from build123d import *

# Parameters (mm, degrees)
BOSS_EXTRUDE1_DEPTH                                  = 50.8
CBORE_FOR_1_4_BINDING_HEAD_MACHINE_SCREW_D           = 6.5278
CBORE_FOR_1_4_BINDING_HEAD_MACHINE_SCREW_CBORE_D     = 14.2875
CBORE_FOR_1_4_BINDING_HEAD_MACHINE_SCREW_CBORE_DEPTH = 3.302
CUT_EXTRUDE1_REACH                                   = 73.186
SKETCH4_R                                            = 3.175


with BuildPart() as part:
    # Sketch1 → Boss-Extrude1 (new body)
    with BuildSketch(Plane(origin=(0, 0, 0), x_dir=(0, 0, -1), z_dir=(1, 0, 0))):
        Polygon((0, 0), (0, 29.972), (39.856315031, 29.972), (39.856315031, 25.3111), (8.106315031, 25.3111), (8.106315031, 4.6609), (39.856315031, 4.6609), (39.856315031, 0), align=None)
    extrude(amount=BOSS_EXTRUDE1_DEPTH)

    # CBORE for 1/4 Binding Head Machine Screw1 (through all)
    with Locations(Plane(origin=(0, 0, -8.106315031), x_dir=(-1, 0, 0), z_dir=(0, 0, -1))):
        with Locations((-12.7, 14.986), (-38.1, 14.986)):
            CounterBoreHole(CBORE_FOR_1_4_BINDING_HEAD_MACHINE_SCREW_D / 2, CBORE_FOR_1_4_BINDING_HEAD_MACHINE_SCREW_CBORE_D / 2, CBORE_FOR_1_4_BINDING_HEAD_MACHINE_SCREW_CBORE_DEPTH)

    # Cut-Extrude1: up to this face of the body (flat: up to its plane)
    cut_extrude1_end = Plane(part.part.faces().sort_by_distance((25.4, 29.972, -19.928157515))[0])
    # Sketch4 → Cut-Extrude1 (cut, up to the picked face)
    with BuildSketch(Plane.XZ, mode=Mode.PRIVATE) as cut_extrude1_sk1:
        with Locations(Location((25.4, -29.497789369, 0), (0, 0, 270))):
            Circle(SKETCH4_R)
    cut_extrude1_tool1 = split(extrude(cut_extrude1_sk1.sketch, amount=-CUT_EXTRUDE1_REACH, mode=Mode.PRIVATE), bisect_by=cut_extrude1_end, keep=Keep.BOTH, mode=Mode.PRIVATE)
    # Sketch4 → Cut-Extrude1 (cut, up to the picked face)
    with BuildSketch(Plane.XZ, mode=Mode.PRIVATE) as cut_extrude1_sk2:
        with BuildLine():
            Line((0, 0), (16.880765903, -33.757868641))
            ThreePointArc((16.880765903, -33.757868641), (25.4, -39.022789369), (33.919234097, -33.757868641))
            Line((33.919234097, -33.757868641), (50.8, 0))
            Line((50.8, 0), (50.8, -39.856315031))
            Line((50.8, -39.856315031), (0, -39.856315031))
            Line((0, -39.856315031), (0, 0))
        make_face()
    cut_extrude1_tool2 = split(extrude(cut_extrude1_sk2.sketch, amount=-CUT_EXTRUDE1_REACH, mode=Mode.PRIVATE), bisect_by=cut_extrude1_end, keep=Keep.BOTH, mode=Mode.PRIVATE)
    add(cut_extrude1_tool1.solids().sort_by(Axis((25.4, 0, -29.497789), (0, 1, 0)))[0], mode=Mode.SUBTRACT)
    add(cut_extrude1_tool2.solids().sort_by(Axis((7.862872, 0, -17.167721), (0, 1, 0)))[0], mode=Mode.SUBTRACT)


solid = part.part
Design review of the part built by this model. Coordinates are the model's own, in mm. A direction names the side the tool comes from. Give positions to 0.01 mm unless a question says otherwise; leave off trailing zeros. Loops run counter-clockwise (first coordinate to the right, second up) from the corner with the lowest first, then second, coordinate; pieces in that order, holes last. Notation, with made-up numbers: (37.5, 50.25) -> (47.5, 50.25) arc R13 ccw to (47.5, 72.25) -> close; hole circle Ø3 at (12, -27). An arc over 180 degrees is marked (long way). One line per question, with ' | ' between items. Start each with the question number.
(1) We need section C-C (y = 16). State the section outline as (x, z) points.
(2) Draft analysis for pull direction X (two halves, no side actions). For faces 1 (the face through (47.87, 14.78, -5.86)), 2 (the face through (45.237, 15.3, -6.478)), 3 (the face through (17.97, 19.81, -6.48)), 4 (the face through (25, 25.311, -20)), state which applies: +X half, -X half, draft (parallel to the pull), parting line (faces both ways), or undercut.
(3) For faces 5 (the face through (28.08, 27.61, -31.2)), 6 (the face through (36.6, 11.9, -4.804)), 7 (the face through (25, 15, -8.106)), list the 3-axis set-ups (+Z, -Z, +X, -X, +Y, -Y) from which the entire face can be reached by the end or side of a thin tool; tool diameter is ignored.
(4) We need section D-D (y = 26). State the section outline as (x, z) points (3 decimals).
(5) We need section A-A (z = -32). State the section outline as (x, y) points, and give its area (3 significant figures).
(6) We need section B-B (x = 25.4). State the section outline as (y, z) points.
(7) Insertion check: P1, Ø11.5, axis at x = 39, y = 12, coming from the -Z side; P2, Ø2, axis at x = 10.5, y = 18, coming from the -Z side; P3, Ø4, axis at y = 23, z = -10, coming from the +X side. Each pin has a flat end and moves straight along its axis. Give the tip position at first contact, or say it passes through.
(8) For line 1 (Y direction, x = 12.7, z = -7.1); line 2 (Y direction, x = 12.7, z = -2.55); line 3 (X direction, y = 16.25, z = -2), list the stretches that pass through material, from the lowest coordinate up.
The answers:
1) outline: (0, 0) -> (4.05, -8.11) -> (5.63, -8.11) -> (5.63, -4.8) -> (9.6, -4.8) -> (9.6, 0) -> close; (15.8, -4.8) -> (19.77, -4.8) -> (19.77, -8.11) -> (31.03, -8.11) -> (31.03, -4.8) -> (35, -4.8) -> (35, 0) -> (15.8, 0) -> close; (41.2, -4.8) -> (45.17, -4.8) -> (45.17, -8.11) -> (46.75, -8.11) -> (50.8, 0) -> (41.2, 0) -> close
2) face 1: +X half | face 2: undercut | face 3: undercut | face 4: draft
3) face 5: +Y, -Y | face 6: -Z | face 7: -Z, +X, -X
4) outline: (0, 0) -> (16.881, -33.758) arc R9.525 ccw to (33.919, -33.758) -> (50.8, 0) -> close; hole circle Ø6.35 at (25.4, -29.498)
5) outline: (16, 0) -> (23.45, 0) -> (23.45, 4.66) -> (16, 4.66) -> close; (16, 25.31) -> (23.45, 25.31) -> (23.45, 29.97) -> (16, 29.97) -> close; (27.35, 0) -> (34.8, 0) -> (34.8, 4.66) -> (27.35, 4.66) -> close; (27.35, 25.31) -> (34.8, 25.31) -> (34.8, 29.97) -> (27.35, 29.97) -> close | area: 139 mm^2
6) outline: (0, -39.02) -> (4.66, -39.02) -> (4.66, -32.67) -> (0, -32.67) -> close; (0, -26.32) -> (4.66, -26.32) -> (4.66, -8.11) -> (25.31, -8.11) -> (25.31, -26.32) -> (29.97, -26.32) -> (29.97, 0) -> (0, 0) -> close; (25.31, -39.02) -> (29.97, -39.02) -> (29.97, -32.67) -> (25.31, -32.67) -> close
7) P1: stops at z = -8.11 | P2: stops at z = -4.8 | P3: stops at x = 46.8
8) line 1: y = 0 to 7.84, 22.13 to 29.97 | line 2: y = 0 to 11.72, 18.25 to 29.97 | line 3: x = 1 to 9.69, 15.71 to 35.09, 41.11 to 49.8
